Work out the finished part from the listing and answer in its coordinate system (mm). A direction names the side the tool comes from. Coordinates: 2 decimals unless noted, no trailing zeros. Write each loop counter-clockwise with the first axis right and the second up, starting at its lowest first coordinate (ties: lowest second). Pieces come first, ordered by that corner, then holes. Notation, with made-up numbers: (76.5, 21.25) - (87.5, 21.25) arc R25 ccw to (87.5, 52.25) - close; hole circle Ø1 at (-13.5, 65). An arc over 180 degrees is marked (long way). Use a Markdown table: item, result. Add a question column.
(1) The part is cut by section B-B, the plane z = 0. Give the vertices of the cut face in (x, y).
(2) Find the intervals of material crossed by line 1 (Y direction, x = 1, z = -3); line 2 (X direction, y = 12.75, z = 0); line 3 (X direction, y = 6, z = -0.75), in increasing order. Write a range as from..to.
(3) The part is cut by section C-C, the plane y = 4.5. Give the vertices of the cut face in (x, z).
(4) Given pin 1 Ø2 at (y, z) = (12.5, 1) entering from -X; pin 2 Ø3 at (x, y) = (-1, 5) entering from -Z; pin 3 Ø1.5 at (y, z) = (3, -2) entering from -X, each flat-ended and moving along its own axis, determine where each tip first touches the part or whether it passes through.
(5) A tool of negligible diameter and unlimited length cuts with its end or side. For faces 1 (the face through (0.676, 7.801, 2.146)), 2 (the face through (0, 15, 0)), from which of +Z, -Z, +X, -X, +Y, -Y can it reach the whole face along a straight path? Write none if from no direction.
(6) The part is cut by section A-A, the plane x = 0. Give the vertices of the cut face in (y, z), then the cut area to 3 significant figures.
from build123d import *

# Parameters (mm, degrees)
SKETCH2_R           = 2.25
BOSS_EXTRUDE1_DEPTH = 15
BOSS_EXTRUDE2_START = -2
SKETCH2_3_R         = 3.25
SKETCH2_3_R_2       = 2.25
BOSS_EXTRUDE2_DEPTH = 2
FILLET1_R           = 0.8


with BuildPart() as part:
    # Sketch2 → Boss-Extrude1 (new body)
    with BuildSketch(Plane(origin=(0, 0, 0), x_dir=(1, 0, 0), z_dir=(0, 1, 0))):
        with Locations(Location((0, 0, 0), (0, 0, 270))):
            Circle(SKETCH2_R)
    extrude(amount=BOSS_EXTRUDE1_DEPTH)

    # Sketch2_3 → Boss-Extrude2 (add)
    # profile 1 of 2: a face of its own
    with BuildSketch(Plane(origin=(0, 0, 0), x_dir=(1, 0, 0), z_dir=(0, 1, 0)).offset(BOSS_EXTRUDE2_START)):
        with Locations(Location((0, 0, 0), (0, 0, 270))):
            Circle(SKETCH2_3_R)
        with Locations(Location((0, 0, 0), (0, 0, 270))):
            Circle(SKETCH2_3_R_2, mode=Mode.SUBTRACT)
    # profile 2 of 2: a face of its own
    with BuildSketch(Plane(origin=(0, 0, 0), x_dir=(1, 0, 0), z_dir=(0, 1, 0)).offset(BOSS_EXTRUDE2_START)):
        with Locations(Location((0, 0, 0), (0, 0, 270))):
            Circle(SKETCH2_3_R_2)
    extrude(amount=BOSS_EXTRUDE2_DEPTH)

    # Fillet1
    fillet1_edges = [part.edges().sort_by_distance(p)[0] for p in [
        (0, 0, -2.25),
    ]]
    fillet(fillet1_edges, radius=FILLET1_R)


solid = part.part
Model answer:
| question | item | result |
|---|---|---|
| 1 | outline | (-3.25, -2) - (3.25, -2) - (3.25, 0) - (3.05, 0) arc R0.8 cw to (2.25, 0.8) - (2.25, 15) - (-2.25, 15) - (-2.25, 0.8) arc R0.8 cw to (-3.05, 0) - (-3.25, 0) - close |
| 2 | line 1 | -2..0 |
| 2 | line 2 | -2.25..2.25 |
| 2 | line 3 | -2.12..2.12 |
| 3 | outline | circle Ø4.5 at (0, 0) |
| 4 | pin 1 | x = -2.25 |
| 4 | pin 2 | z = -2.25 |
| 4 | pin 3 | x = -1.87 |
| 5 | face 1 | +Y |
| 5 | face 2 | +Z, -Z, +X, -X, +Y |
| 6 | outline | (-2, -3.25) - (0, -3.25) - (0, -3.05) arc R0.8 cw to (0.8, -2.25) - (15, -2.25) - (15, 2.25) - (0.8, 2.25) arc R0.8 cw to (0, 3.05) - (0, 3.25) - (-2, 3.25) - close |
| 6 | area | 80.8 mm^2 |
